Source: CAD feature listing. Evaluate the final solid. Frame: model axes, mm. A direction names the side the tool comes from. Give positions to 0.01 mm unless a question says otherwise; leave off trailing zeros. Write each loop counter-clockwise with the first axis right and the second up, starting at its lowest first coordinate (ties: lowest second). Pieces come first, ordered by that corner, then holes. Notation, with made-up numbers: M 2.5,57 L 50.5,57 A12 ccw 50.5,75 Z; hole C 15,-19 d6. An arc over 180 degrees is marked long. Return JSON: item names as keys, results as strings.
```python
from build123d import *

# Parameters (mm, degrees)
BOSS_EXTRUDE1_DEPTH     = 50
CUT_EXTRUDE1_DEPTH      = 94.512708955
CUT_EXTRUDE1_DEPTH_BACK = 94.512708955
SKETCH2_R               = 16
SKETCH3_R               = 16
CUT_EXTRUDE2_DEPTH      = 93.736184955
TAP_DRILL_FOR_M3_TAP1_D = 2.5
TAP_DRILL_FOR_M3_TAP2_D = 2.5
CHAMFER1_SIZE           = 2
BOSS_EXTRUDE2_DEPTH     = 50
FILLET1_R               = 2
FILLET2_R               = 5
M3_CLEARANCE_HOLE1_D    = 3.6


with BuildPart() as part:
    # Sketch1 → Boss-Extrude1 (new body)
    with BuildSketch(Plane(origin=(0, 0, 0), x_dir=(1, 0, 0), z_dir=(0, 1, 0))):
        Polygon((-12, -43.458333333), (-6, -43.458333333), (-6, 6.541666667), (54, 6.541666667), (54, -43.458333333), (60, -43.458333333), (60, 12.541666667), (-12, 12.541666667), align=None)
    extrude(amount=BOSS_EXTRUDE1_DEPTH)

    # Sketch2 → Cut-Extrude1 (cut, two sides: drawn at the far end of the back side and taken through both)
    with BuildSketch(Plane(origin=(-6, 0, 0), x_dir=(0, 0, -1), z_dir=(1, 0, 0)).offset(-CUT_EXTRUDE1_DEPTH_BACK)):
        with Locations((-23.458333333, 25)):
            Circle(SKETCH2_R)
    extrude(amount=CUT_EXTRUDE1_DEPTH + CUT_EXTRUDE1_DEPTH_BACK, mode=Mode.SUBTRACT)

    # Sketch3 → Cut-Extrude2 (cut, through all)
    with BuildSketch(Plane.XY.offset(-6.541666667)):
        with Locations((24, 25)):
            Circle(SKETCH3_R)
    extrude(amount=-CUT_EXTRUDE2_DEPTH, mode=Mode.SUBTRACT)

    # Tap Drill for M3 Tap1 (through all)
    with Locations(Plane(origin=(60, 0, 0), x_dir=(0, 0, -1), z_dir=(1, 0, 0))):
        with Locations((-39.36823591, 9.090097423), (-39.36823591, 40.909902577), (-7.548430757, 40.909902577), (-7.548430757, 9.090097423)):
            Hole(TAP_DRILL_FOR_M3_TAP1_D / 2)

    # Tap Drill for M3 Tap2 (through all)
    with Locations(Plane(origin=(0, 0, -12.541666667), x_dir=(-1, 0, 0), z_dir=(0, 0, -1))):
        with Locations((-39.909902577, 9.090097423), (-39.909902577, 40.909902577), (-8.090097423, 40.909902577), (-8.090097423, 9.090097423)):
            Hole(TAP_DRILL_FOR_M3_TAP2_D / 2)

    # Chamfer1
    chamfer1_edges = [part.edges().sort_by_distance(p)[0] for p in [
        (54, 25, -6.541666667),
        (-6, 25, -6.541666667),
    ]]
    chamfer(chamfer1_edges, length=CHAMFER1_SIZE)

    # Sketch9 → Boss-Extrude2 (add)
    with BuildSketch(Plane(origin=(0, 50, 0), x_dir=(1, 0, 0), z_dir=(0, 1, 0))):
        Polygon((-12, 0.541666667), (-17, 0.541666667), (-17, 17.541666667), (0, 17.541666667), (0, 12.541666667), (-12, 12.541666667), align=None)
        Polygon((65, 17.541666667), (65, 0.541666667), (60, 0.541666667), (60, 12.541666667), (48, 12.541666667), (48, 17.541666667), align=None)
    extrude(amount=-BOSS_EXTRUDE2_DEPTH)

    # Fillet1
    fillet1_edges = [part.edges().sort_by_distance(p)[0] for p in [
        (-12, 25, -0.541666667),
        (-17, 25, -0.541666667),
        (0, 25, -17.541666667),
        (0, 25, -12.541666667),
        (48, 25, -17.541666667),
        (65, 25, -0.541666667),
        (60, 25, -0.541666667),
        (48, 25, -12.541666667),
    ]]
    fillet(fillet1_edges, radius=FILLET1_R)

    # Fillet2
    fillet2_edges = [part.edges().sort_by_distance(p)[0] for p in [
        (-17, 25, -17.541666667),
        (65, 25, -17.541666667),
    ]]
    fillet(fillet2_edges, radius=FILLET2_R)

    # M3 Clearance Hole1 (through all)
    with Locations(Plane(origin=(0, 50, 0), x_dir=(1, 0, 0), z_dir=(0, 1, 0))):
        with Locations((-9, 9.541666667), (57, 9.541666667)):
            Hole(M3_CLEARANCE_HOLE1_D / 2)


solid = part.part
```
1) Cut plane B-B, the plane z = 10. Return the cut outline in (x, y).
Numbers:
{"outline": "M -12,0 L -6,0 L -6,16.35 L -12,16.35 Z; M -12,33.65 L -6,33.65 L -6,50 L -12,50 Z; M 54,0 L 60,0 L 60,16.35 L 54,16.35 Z; M 54,33.65 L 60,33.65 L 60,50 L 54,50 Z"}
2) Contact query for flat-ended pins moving along their axis: pin 1 Ø2 at (x, y) = (39.91, 40.91) entering from +Z; pin 2 Ø14.5 at (y, z) = (15, 23) entering from -X; pin 3 Ø3 at (y, z) = (9.09, 39.37) entering from +X; pin 4 Ø2 at (x, y) = (47.5, 6) entering from +Z. Output: stop coordinate, or through.
Numbers:
{"pin 1": "passes through", "pin 2": "stops at x = -12", "pin 3": "stops at x = 60", "pin 4": "stops at z = -6.54"}
3) Cut plane A-A, the plane x = 57. Return the cut outline in (y, z).
Numbers:
{"outline": "M 0,-17.54 L 50,-17.54 L 50,-11.34 L 0,-11.34 Z; M 0,-7.74 L 50,-7.74 L 50,43.46 L 0,43.46 Z; hole C 9.09,7.55 d2.5; hole C 9.09,39.37 d2.5; hole C 25,23.46 d32; hole C 40.91,7.55 d2.5; hole C 40.91,39.37 d2.5"}
4) Line query: line 1 (Y direction, x = 24, z = -8); line 2 (X direction, y = 42, z = 6.5); line 3 (Z direction, x = 7.5, y = 18). Output: solid intervals per line, ascending. Write a range as [from, to].
Numbers:
{"line 1": "y = [0, 9], [41, 50]", "line 2": "x = [-12, -6], [54, 60]", "line 3": "z = [-12.54, -6.54]"}
5) Draft query along X for faces 1 (the face through (56.96, 18.87, 8.68)), 2 (the face through (63.496, 24.65, -16.116)), 3 (the face through (-7.57, 24.65, -8.45)). Return one class per face: released by +X, released by -X, zero draft, split by the parting line, or undercut.
Numbers:
{"face 1": "zero draft", "face 2": "released by +X", "face 3": "undercut"}
6) Set-up query: faces 4 (the face through (-9, 25, 43.458)), 5 (the face through (-4.986, 24.65, -5.556)), 6 (the face through (48.57, 24.65, -16.94)). Return all of +Z, -Z, +X, -X, +Y, -Y with unobstructed straight access to the full face (end or side cutting, diameter ignored); none if empty.
Numbers:
{"face 4": "+Z, +X, -X, +Y, -Y", "face 5": "+Z, +Y, -Y", "face 6": "-Z, +Y, -Y"}
7) Cut plane C-C, the plane x = 24. Return the cut outline in (y, z), then the cut area to 3 significant figures.
Numbers:
{"outline": "M 0,-12.54 L 9,-12.54 L 9,-6.54 L 0,-6.54 Z; M 41,-12.54 L 50,-12.54 L 50,-6.54 L 41,-6.54 Z", "area": "108 mm²"}
8) Cut plane D-D, the plane y = 19.5. Give the number of separate pieces and of enclosed holes in the cut face, then the cut area to 3 significant figures.
Numbers:
{"separate pieces": "4", "enclosed holes": "2", "area": "754 mm²"}
